The listing builds one solid part. Answer for the finished solid, in the listing's coordinates (mm). Face numbers are marked on the shaded views. A direction names the side the tool comes from. Round coordinates to 2 decimals unless told otherwise and drop trailing zeros. Write each loop counter-clockwise with the first axis right and the second up, starting at its lowest first coordinate (ties: lowest second). Pieces come first, ordered by that corner, then holes. Notation, with made-up numbers: M 0.5,60 L 9.5,60 A14 cw 9.5,72 Z; hole C -32,54 d5. An arc over 180 degrees is marked long. One line per item, written item: value. Start each with the question number.
(1) Section C-C (y = 9) is taken. Determine the outline of the cut face in (x, z), plus the area to 3 significant figures.
(2) Section A-A (x = 15) is taken. Determine the outline of the cut face in (y, z).
(3) Section B-B (z = -24.5) is taken. Determine the outline of the cut face in (x, y).
(4) For the marked faces 1 and 2, determine the directions among +Z, -Z, +X, -X, +Y, -Y from which every point of the face is accessible in a straight line to the end or side of a thin tool.
(5) Given P1, Ø12, axis at x = 11.5, y = 22.5, coming from the -Z side; P2, Ø5, axis at x = 5.5, y = -31, coming from the +Z side; P3, Ø3, axis at x = 15, z = 107, coming from the +Y side; P4, Ø17, axis at x = 15, z = -30.54, coming from the +Y side, each flat-ended and moving along its own axis, determine where each tip first touches the part or whether it passes through.
(6) Section D-D (y = -35) is taken. Determine the outline of the cut face in (x, z).
(7) Consider probe 1 along Z at (x, y) = (15, -37.75); probe 2 along Y at (x, z) = (23.75, -12); probe 3 along Z at (x, y) = (22.75, 29.5). Determine where each line is inside the solid, lowest interval first.
(8) For a pull along Y with two mould halves and no side action, classify the marked faces 3, 4, 5 and 6 as released by +Y, released by -Y, zero draft, split by the parting line, or undercut.
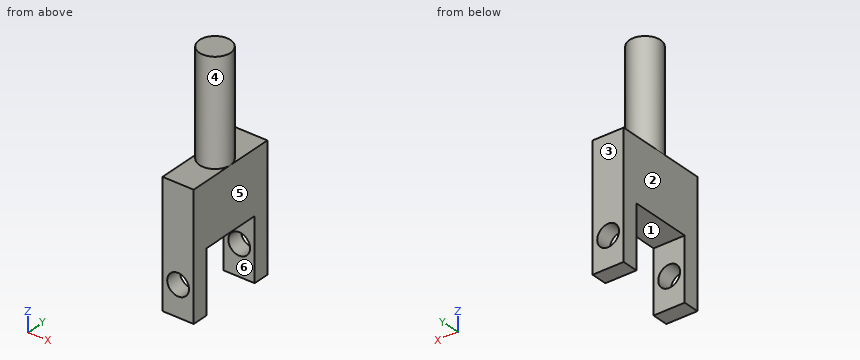
```python
from build123d import *

# Parameters (mm, degrees)
F0_W     = 90.468154
F0_H     = 119.692906
F1_DEPTH = 30
F2_W     = 59.248916
F2_H     = 119.692907
F3_DEPTH = 30
F4_R     = 15
F5_DEPTH = 100
F6_R     = 10.508177
F7_DEPTH = 100


with BuildPart() as f1:
    # F0 (on Right) → F1 (new body)
    with BuildSketch(Plane.YZ):
        Rectangle(F0_W, F0_H)
    extrude(amount=F1_DEPTH)

    # F2 (on face) → F3 (cut)
    with BuildSketch(Plane.YZ.offset(30)):
        with Locations((0, -59.846453)):
            Rectangle(F2_W, F2_H)
    extrude(amount=-F3_DEPTH, mode=Mode.SUBTRACT)

    # F4 (on face) → F5 (join)
    with BuildSketch(Plane.XY.offset(59.846453)):
        with Locations((15, 0)):
            Circle(F4_R)
    extrude(amount=F5_DEPTH)

    # F6 (on face) → F7 (cut)
    with BuildSketch(Plane.XZ.offset(45.234077)):
        with Locations((15, -30.535292)):
            Circle(F6_R)
    extrude(amount=-F7_DEPTH, mode=Mode.SUBTRACT)


solid = f1.part
```
Recorded:
1. outline: M 0,0 L 30,0 L 30,59.85 L 27,59.85 L 27,159.85 L 3,159.85 L 3,59.85 L 0,59.85 Z
1. area: 4,200 mm2
2. outline: M -45.23,-59.85 L -29.62,-59.85 L -29.62,-41.04 L -45.23,-41.04 Z; M -45.23,-20.03 L -29.62,-20.03 L -29.62,0 L 29.62,0 L 29.62,-20.03 L 45.23,-20.03 L 45.23,59.85 L 15,59.85 L 15,159.85 L -15,159.85 L -15,59.85 L -45.23,59.85 Z; M 29.62,-59.85 L 45.23,-59.85 L 45.23,-41.04 L 29.62,-41.04 Z
3. outline: M 0,-45.23 L 6.4,-45.23 L 6.4,-29.62 L 0,-29.62 Z; M 0,29.62 L 6.4,29.62 L 6.4,45.23 L 0,45.23 Z; M 23.6,-45.23 L 30,-45.23 L 30,-29.62 L 23.6,-29.62 Z; M 23.6,29.62 L 30,29.62 L 30,45.23 L 23.6,45.23 Z
4. face 1: -Z, +X, -X
4. face 2: +Z, -Z, -X, +Y, -Y
5. P1: stops at z = 0
5. P2: stops at z = 59.85
5. P3: stops at y = 15
5. P4: passes through
6. outline: M 0,-59.85 L 30,-59.85 L 30,59.85 L 0,59.85 Z; hole C 15,-30.54 d21.02
7. probe 1: z = -59.85 to -41.04, -20.03 to 59.85
7. probe 2: y = -45.23 to -29.62, 29.62 to 45.23
7. probe 3: z = 0 to 59.85
8. face 3: released by +Y
8. face 4: split by the parting line
8. face 5: zero draft
8. face 6: undercut
